Geometry check sheet. Reference: the model listing, model coordinates, mm. A direction names the side the tool comes from. Round coordinates to 2 decimals unless told otherwise and drop trailing zeros. Write each loop counter-clockwise with the first axis right and the second up, starting at its lowest first coordinate (ties: lowest second). Pieces come first, ordered by that corner, then holes.
Autodesk Inventor part; units mm, degrees
ref_plane "YZ Plane" through (0, 0, 0) normal (1, 0, 0) x (0, 1, 0)
ref_plane "XZ Plane" through (0, 0, 0) normal (0, 1, 0) x (-1, 0, 0)
ref_plane "XY Plane" through (0, 0, 0) normal (0, 0, 1) x (1, 0, 0)
sketch "Sketch1" plane through (0, 0, 0) normal (0, 1, 0) x (-1, 0, 0)
  line L0 (-83.5, 139.5) -> (83.5, 139.5)
  line L1 (83.5, 139.5) -> (83.5, -139.5)
  line L2 (83.5, -139.5) -> (-83.5, -139.5)
  line L3 (-83.5, -139.5) -> (-83.5, 139.5)
  line L4 (-83.5, 139.5) -> (83.5, -139.5) construction
  line L5 (83.5, 139.5) -> (-83.5, -139.5) construction
  point P0 (0, 0)
  dimension "d0" = 167
  dimension "d1" = 279
extrude "Extrusion1" add sketch "Sketch1" along normal blind 80
sketch "Sketch2" plane through (0, 80, 0) normal (0, 1, 0) x (1, 0, 0)
  line L0 (71.5, -119.5) -> (-71.5, -119.5)
  line L1 (-73.5, -117.5) -> (-73.5, 117.5)
  line L2 (-71.5, 119.5) -> (71.5, 119.5)
  line L3 (73.5, 117.5) -> (73.5, -117.5)
  line L4 (73.5, -119.5) -> (-73.5, 119.5) construction
  line L5 (-73.5, -119.5) -> (73.5, 119.5) construction
  arc A0 (-73.5, -117.5) -> (-71.5, -119.5) centre (-71.5, -117.5) ccw
  arc A1 (-71.5, 119.5) -> (-73.5, 117.5) centre (-71.5, 117.5) ccw
  arc A2 (73.5, 117.5) -> (71.5, 119.5) centre (71.5, 117.5) ccw
  arc A3 (71.5, -119.5) -> (73.5, -117.5) centre (71.5, -117.5) ccw
  point P0 (0, 0)
  dimension "d4" = 147
  dimension "d5" = 239
  dimension "d6" = 2
extrude "Extrusion2" cut sketch "Sketch2" against normal blind 1.1
sketch "Sketch3" plane through (0, 78.9, 0) normal (0, 1, 0) x (1, 0, 0)
  line L0 (-73.5, -117.5) -> (-73.5, 117.5)
  line L1 (71.5, -119.5) -> (-71.5, -119.5)
  line L2 (-72.25, -117.83) -> (72.25, -117.83)
  line L3 (72.25, -117.83) -> (72.25, 112.27)
  line L4 (72.25, 112.27) -> (-72.25, 112.27)
  line L5 (-72.25, 112.27) -> (-72.25, -117.83)
  point P0 (0, 0)
  dimension "d9" = 1.25
  dimension "d10" = 1.67
  dimension "d11" = 144.5
  dimension "d12" = 230.1
extrude "Extrusion3" cut sketch "Sketch3" against normal blind 73.9
sketch "Sketch4" plane through (0, 5, 0) normal (0, 1, 0) x (1, 0, 0)
  circle A0 centre (-66.5, -111.83) radius 2
  line L0 (72.25, -117.83) -> (-72.25, -117.83)
  line L1 (-72.25, -117.83) -> (-72.25, 112.27)
  circle A1 centre (66.5, -111.83) radius 2
  line L2 (72.25, 112.27) -> (72.25, -117.83)
  circle A2 centre (-66.5, 106.27) radius 2
  line L3 (-72.25, 112.27) -> (72.25, 112.27)
  circle A3 centre (66.5, 106.27) radius 2
  point P0 (0, 0)
  dimension "d15" = 4
  dimension "d16" = 6
  dimension "d17" = 5.75
  dimension "d18" = 4
  dimension "d19" = 6
  dimension "d20" = 5.75
  dimension "d21" = 4
  dimension "d22" = 5.75
  dimension "d23" = 6
  dimension "d24" = 4
  dimension "d25" = 6
  dimension "d26" = 5.75
extrude "Extrusion4" add sketch "Sketch4" along normal blind 73.9 contours A0 | A1 | A2 | A3
sketch "Sketch5" plane through (0, 5, 0) normal (0, 1, 0) x (1, 0, 0)
  circle A0 centre (-66.5, -111.83) radius 2
  circle A1 centre (-66.5, -111.83) radius 1.25
  circle A2 centre (-66.5, 106.27) radius 2
  circle A3 centre (-66.5, 106.27) radius 1.25
  circle A4 centre (66.5, 106.27) radius 2
  circle A5 centre (66.5, 106.27) radius 1.25
  circle A6 centre (66.5, -111.83) radius 1.25
  point P0 (0, 0)
  dimension "d29" = 2.5
  dimension "d30" = 2.5
  dimension "d31" = 2.5
  dimension "d32" = 2.5
extrude "Extrusion5" cut sketch "Sketch5" along normal blind 73.9 and the other way blind 5 contours A1 | A3 | A5 | A6
sketch "Sketch6" plane through (0, 0, 0) normal (0, -1, 0) x (1, 0, 0)
  circle A0 centre (-66.5, -106.27) radius 1.25
  circle A1 centre (-66.5, -106.27) radius 1.75
  circle A2 centre (-66.5, 111.83) radius 1.25
  circle A3 centre (-66.5, 111.83) radius 1.75
  circle A4 centre (66.5, 111.83) radius 1.25
  circle A5 centre (66.5, 111.83) radius 1.75
  circle A6 centre (66.5, -106.27) radius 1.25
  circle A7 centre (66.5, -106.27) radius 1.75
  point P0 (0, 0)
  dimension "d37" = 3.5
  dimension "d38" = 3.5
  dimension "d39" = 3.5
  dimension "d40" = 3.5
extrude "Extrusion6" cut sketch "Sketch6" against normal blind 76.9 contours A0 | A1 | A2 | A3 | A4 | A5 | A6 | A7
properties part number "Enclosure"
1. Release check for a two-part mould opening along X. For faces 3 (the face through (1, 0, 2)), 4 (the face through (-1, 42, 117.83)), 5 (the face through (-83.5, 39, 2)) record: +X half, -X half, draft (parallel to the pull), parting line (faces both ways), or undercut.
2. Depth check by flat-ended pin: pin 1 Ø4.5 at (x, z) = (-66.5, -106.27) entering from +Y; pin 2 Ø1 at (x, z) = (-12.5, 42.5) entering from +Y. Enter the tip coordinate at first touch or a pass-through.
3. Scan lines: line 1 along Z through (x, y) = (-66.5, 78); line 2 along X through (y, z) = (35.5, -106.27); line 3 along Z through (x, y) = (-66.5, 37). Record each from-to range of solid material in increasing order.
4. Access from +Z, -Z, +X, -X, +Y, -Y to the whole of each face (thin tool, end or side, straight path). Record for faces 1 (the face through (-1, 5, 1)), 2 (the face through (75, 80, 1)).
5. Section check C-C (z = -74.5). Record the cut outline in (x, y).
6. Section check B-B (x = 53). Record the cut outline in (y, z), plus the area to 3 significant figures.
7. Section check A-A (y = 49.5). State how many separate pieces and enclosed holes the cut face has, plus the area to 3 significant figures.
Results below:
1. face 3: draft
1. face 4: undercut
1. face 5: -X half
2. pin 1: stops at y = 78.9
2. pin 2: stops at y = 5
3. line 1: z = -139.5 to -112.27, -108.27 to -107.52, -105.02 to -104.27, 109.83 to 110.58, 113.08 to 113.83, 117.83 to 139.5
3. line 2: x = -83.5 to -72.25, -68.5 to -68.25, -64.75 to -64.5, 64.5 to 64.75, 68.25 to 68.5, 72.25 to 83.5
3. line 3: z = -139.5 to -112.27, -108.27 to -108.02, -104.52 to -104.27, 109.83 to 110.08, 113.58 to 113.83, 117.83 to 139.5
4. face 1: +Y
4. face 2: +Z, -Z, +X, -X, +Y
5. outline: (-83.5, 0) - (83.5, 0) - (83.5, 80) - (73.5, 80) - (73.5, 78.9) - (72.25, 78.9) - (72.25, 5) - (-72.25, 5) - (-72.25, 78.9) - (-73.5, 78.9) - (-73.5, 80) - (-83.5, 80) - close
6. outline: (0, -139.5) - (80, -139.5) - (80, -119.5) - (78.9, -119.5) - (78.9, -112.27) - (5, -112.27) - (5, 117.83) - (78.9, 117.83) - (78.9, 119.5) - (80, 119.5) - (80, 139.5) - (0, 139.5) - close
6. area: 5,050 mm2
7. separate pieces: 5
7. enclosed holes: 5
7. area: 13,400 mm2
